from build123d import *

# Parameters (mm, degrees)
SKETCH009_W        = 106
SKETCH009_H        = 22
PAD003_DEPTH       = 3
POCKET003002_DEPTH = 219.602016
SKETCH001007_R     = 1.5
POCKET003007_DEPTH = 3.001


with BuildPart() as part:
    # Sketch009 → Pad003 (new body)
    with BuildSketch(Plane.XY):
        with Locations((0, -101)):
            Rectangle(SKETCH009_W, SKETCH009_H)
    extrude(amount=PAD003_DEPTH)

    # Sketch001001 → Pocket003002 (cut, through all)
    with BuildSketch(Plane.XY.offset(3)):
        with BuildLine():
            Line((-50, -106), (-50, -112))
            Line((-50, -112), (-53, -112))
            Line((-53, -112), (-53, -106))
            Line((-53, -106), (-51.923996, -106))
            ThreePointArc((-50, -106), (-50.961998, -105.038002), (-51.923996, -106))
        make_face()
        with BuildLine():
            Line((-4, -90), (-53, -90))
            Line((-53, -90), (-53, -98))
            Line((-51.654504, -98), (-53, -98))
            ThreePointArc((-51.654504, -98), (-50.827252, -98.827252), (-50, -98))
            Line((-50, -98), (-50, -93))
            Line((-50, -93), (-4, -93))
            ThreePointArc((-4, -93), (-3.362141, -92.362141), (-4, -91.724282))
            Line((-4, -90), (-4, -91.724282))
        make_face()
    pocket003002 = extrude(amount=-POCKET003002_DEPTH, mode=Mode.SUBTRACT)

    # Mirrored002: Pocket003002 across Sketch001001 V_Axis
    add(pocket003002.mirror(Plane(origin=(0, 0, 3), x_dir=(0, 0, 1), z_dir=(1, 0, 0))), mode=Mode.SUBTRACT)

    # Sketch001007 → Pocket003007 (cut, through all)
    with BuildSketch(Plane.XY.offset(3)):
        with Locations((0, -102.207499)):
            Circle(SKETCH001007_R)
    extrude(amount=-POCKET003007_DEPTH, mode=Mode.SUBTRACT)


solid = part.part
Build history of the part. All positions in model axes, mm. A direction names the side the tool comes from. Coordinates: 2 decimals unless noted, no trailing zeros. Order: outer loops, then holes, each group sorted by start corner. A loop starts at its lowest first (then second) coordinate and runs counter-clockwise, first axis right, second up. Notation, with made-up numbers: M 21.5,45.5 L 68.5,45.5 A27 ccw 68.5,63.5 Z; hole C -6.75,54.5 d3. An arc over 180 degrees is marked long. One line per question, with ' | ' between items. Start each with the question number.
Q1. Probe L1, parallel to Y at x = 0, z = 2.3; L2, parallel to X at y = -98.75, z = 1.3; L3, parallel to X at y = -98.5, z = 2.6. List the from-to ranges inside material, lowest first. Write a range as from..to.
Q2. 3-axis set-ups, long thin cutter, end or side, ignore diameter. For faces 1 (the face through (-50, -96, 2)), 2 (the face through (50, -96, 2)), 3 (the face through (50, -109, 2)), 4 (the face through (-50.845, -98.827, 1.521)): which of +Z, -Z, +X, -X, +Y, -Y reach the whole face in a straight line?
Q3. Flat gauge pins, fed straight in: pin 1 Ø3 at (x, y) = (-33.5, -98) entering from -Z; pin 2 Ø0.9 at (y, z) = (-108.5, 1) entering from +X; pin 3 Ø1.4 at (y, z) = (-90.5, 2) entering from +X; pin 4 Ø0.9 at (x, z) = (-20, 1.5) entering from +Y. Where does each tip first touch, or does it go through?
Q4. Saw through at C-C (y = -94). List the corners of the cut face in (x, z).
Q5. Saw through at B-B (z = 1.45). List the corners of the cut face in (x, y), then the cut area to 3 significant figures.
Q6. Saw through at D-D (x = 21.5). List the corners of the cut face in (y, z).
Q7. Saw through at A-A (x = 0). List the corners of the cut face in (y, z), then the cut area to 3 significant figures.
Check values:
1) L1: y = -112..-103.71, -100.71..-90 | L2: x = -53..-51.18, -50.48..50.48, 51.18..53 | L3: x = -53..-51.49, -50.17..50.17, 51.49..53
2) face 1: +Z, -Z, -X, +Y | face 2: +Z, -Z, +X, +Y | face 3: +Z, -Z, +X, -Y | face 4: +Z, -Z, +Y
3) pin 1: stops at z = 0 | pin 2: stops at x = 50 | pin 3: stops at x = 4 | pin 4: stops at y = -93
4) outline: M -50,0 L 50,0 L 50,3 L -50,3 Z
5) outline: M -53,-106 L -51.92,-106 A0.96 cw -50,-106 L -50,-112 L 50,-112 L 50,-106 A0.96 cw 51.92,-106 L 53,-106 L 53,-98 L 51.65,-98 A0.83 cw 50,-98 L 50,-93 L 4,-93 A0.64 cw 4,-91.72 L 4,-90 L -4,-90 L -4,-91.72 A0.64 cw -4,-93 L -50,-93 L -50,-98 A0.83 cw -51.65,-98 L -53,-98 Z; hole C 0,-102.21 d3 | area: 1,960 mm2
6) outline: M -112,0 L -93,0 L -93,3 L -112,3 Z
7) outline: M -112,0 L -103.71,0 L -103.71,3 L -112,3 Z; M -100.71,0 L -90,0 L -90,3 L -100.71,3 Z | area: 57.0 mm2
